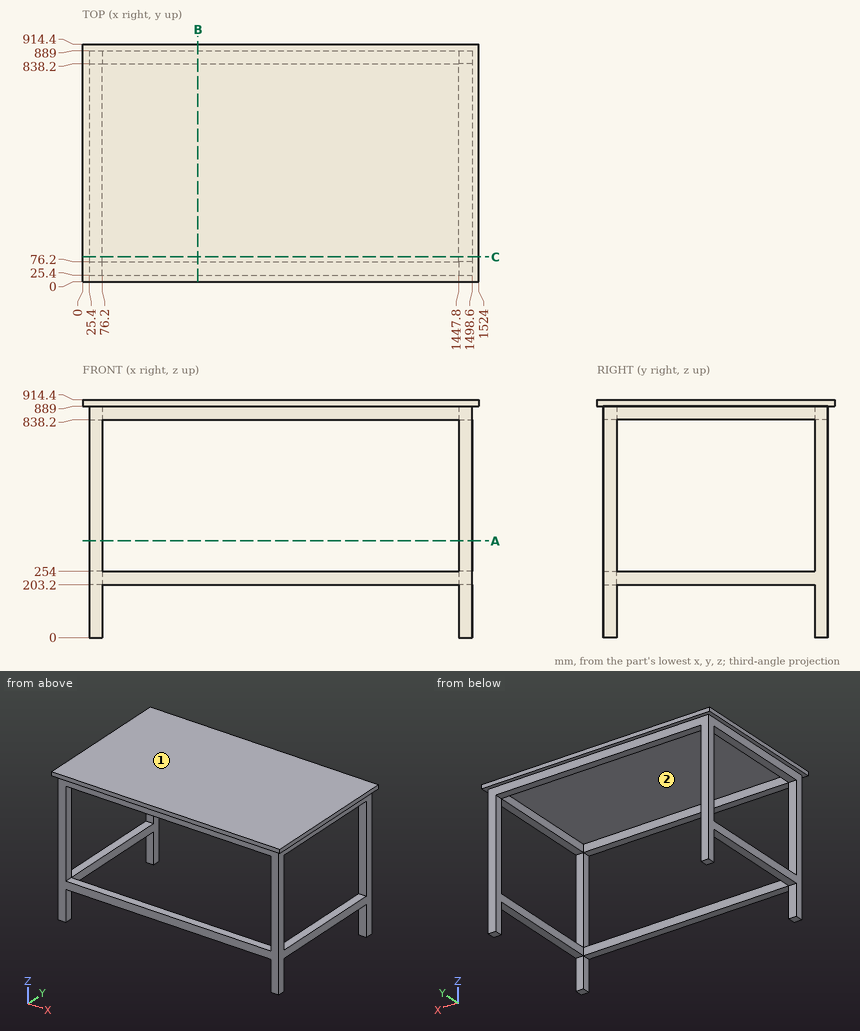
Geometry check sheet. Reference: drawing and pictorial views, mm from the part's lowest x, y, z. Round coordinates to 2 decimals unless told otherwise and drop trailing zeros. Write each loop counter-clockwise with the first axis right and the second up, starting at its lowest first coordinate (ties: lowest second). Pieces come first, ordered by that corner, then holes.
1. Gauge pin test, flat ends, axial feed: P1, Ø4, axis at x = 374.5, y = 214, coming from the -Z side; P2, Ø15, axis at y = 47.5, z = 84, coming from the +X side; P3, Ø4, axis at x = 579.5, z = 221.5, coming from the +Y side. Record the tip position at first contact, or that the pin passes through.
2. Section check A-A on z = 372. Enter the section's corners in (x, y).
3. Section check B-B on x = 444. Enter the section's corners in (y, z), plus the area to 3 significant figures.
4. Section check C-C on y = 96. Enter the section's corners in (x, z).
5. Scan lines: L1, parallel to X at y = 821, z = 226.5; L2, parallel to Z at x = 1184.5, y = 38.5; L3, parallel to Z at x = 1366.5, y = 495. Record each from-to range of solid material in increasing order.
6. Draft check along X on the marked faces 1 and 2. Enter one of: +X half, -X half, draft (parallel to the pull), parting line (faces both ways), or undercut.
Answer:
1. P1: stops at z = 889
1. P2: stops at x = 1498.6
1. P3: stops at y = 76.2
2. outline: (25.4, 25.4) - (76.2, 25.4) - (76.2, 76.2) - (25.4, 76.2) - close; (25.4, 838.2) - (76.2, 838.2) - (76.2, 889) - (25.4, 889) - close; (1447.8, 25.4) - (1498.6, 25.4) - (1498.6, 76.2) - (1447.8, 76.2) - close; (1447.8, 838.2) - (1498.6, 838.2) - (1498.6, 889) - (1447.8, 889) - close
3. outline: (0, 889) - (25.4, 889) - (25.4, 838.2) - (76.2, 838.2) - (76.2, 889) - (838.2, 889) - (838.2, 838.2) - (889, 838.2) - (889, 889) - (914.4, 889) - (914.4, 914.4) - (0, 914.4) - close; (25.4, 203.2) - (76.2, 203.2) - (76.2, 254) - (25.4, 254) - close
3. area: 31,000 mm2
4. outline: (0, 889) - (25.4, 889) - (25.4, 838.2) - (76.2, 838.2) - (76.2, 889) - (1447.8, 889) - (1447.8, 838.2) - (1498.6, 838.2) - (1498.6, 889) - (1524, 889) - (1524, 914.4) - (0, 914.4) - close; (25.4, 203.2) - (76.2, 203.2) - (76.2, 254) - (25.4, 254) - close; (1447.8, 203.2) - (1498.6, 203.2) - (1498.6, 254) - (1447.8, 254) - close
5. L1: x = 25.4 to 76.2, 1447.8 to 1498.6
5. L2: z = 203.2 to 254, 838.2 to 914.4
5. L3: z = 889 to 914.4
6. face 1: draft
6. face 2: undercut
